Could you check a few things on this model? Use its own coordinates, in mm. A direction names the side the tool comes from. Give positions to 0.01 mm unless a question says otherwise; leave off trailing zeros. Order: outer loops, then holes, each group sorted by start corner. A loop starts at its lowest first (then second) coordinate and runs counter-clockwise, first axis right, second up. Notation, with made-up numbers: M -27.5,-3 L 2.5,-3 A22 cw 2.5,19 Z; hole C -37.5,-35.75 d11. An arc over 180 degrees is marked long. Answer in a Markdown table with one row per item. Add a question column.
```python
from build123d import *

# Parameters (mm, degrees)
F0_W      = 57.15
F0_H      = 88.9
F1_DEPTH  = 3.96875
F3_DEPTH  = 7.9375
F5_DEPTH  = 7.9375
F7_DEPTH  = 28.575
F8_R      = 9.92251
F9_DEPTH  = 25.4
F10_R     = 9.92251
F11_DEPTH = 25.4
F13_DEPTH = 7.9375
F14_R     = 10.3251
F15_DEPTH = 25.4
F16_DEPTH = 25.4
F18_DEPTH = 7.9375


with BuildPart() as f1:
    # F0 (on Front) → F1 (new body, symmetric)
    with BuildSketch(Plane.XZ):
        with Locations((28.575, 44.45)):
            Rectangle(F0_W, F0_H)
    extrude(amount=F1_DEPTH, both=True)

    # F2 (on face) → F3 (join)
    with BuildSketch(Plane(origin=(0, 0, 0), x_dir=(1, 0, 0), z_dir=(0, 0, -1))):
        with BuildLine():
            Line((0, 40.48125), (0, -3.96875))
            Line((0, -3.96875), (28.575, -3.96875))
            Line((28.575, -3.96875), (28.575, 40.48125))
            ThreePointArc((28.575, 40.48125), (14.2875, 54.76875), (0, 40.48125))
        make_face()
    extrude(amount=-F3_DEPTH)

    # F4 (on face) → F5 (join)
    with BuildSketch(Plane.XY.offset(88.9)):
        with BuildLine():
            Line((28.575, -40.160799), (28.575, 3.96875))
            Line((28.575, 3.96875), (0, 3.96875))
            Line((0, 3.96875), (0, -40.160799))
            ThreePointArc((0, -40.160799), (14.2875, -54.772343), (28.575, -40.160799))
        make_face()
    extrude(amount=-F5_DEPTH)

    # F6 (on face) → F7 (join)
    with BuildSketch(Plane(origin=(0, 0, 0), x_dir=(0, -1, 0), z_dir=(-1, 0, 0))):
        with BuildLine():
            Line((7.685762, 80.9625), (9.703519, 80.9625))
            ThreePointArc((9.703519, 80.9625), (8.694641, 81.070586), (7.685762, 80.9625))
        make_face()
        with BuildLine():
            ThreePointArc((3.96875, 76.897462), (5.179953, 79.521865), (7.685762, 80.9625))
            Line((7.685762, 80.9625), (3.96875, 80.9625))
            Line((3.96875, 80.9625), (3.96875, 76.897462))
        make_face()
        with BuildLine():
            Line((9.921576, 7.9375), (7.539107, 7.9375))
            ThreePointArc((7.539107, 7.9375), (8.730341, 7.786113), (9.921576, 7.9375))
        make_face()
        with BuildLine():
            ThreePointArc((7.539107, 7.9375), (4.993725, 9.595801), (3.96875, 12.455584))
            Line((3.96875, 12.455584), (3.96875, 7.9375))
            Line((3.96875, 7.9375), (7.539107, 7.9375))
        make_face()
    extrude(amount=-F7_DEPTH)

    # F8 (on face) → F9 (cut)
    with BuildSketch(Plane(origin=(0, 0, 0), x_dir=(1, 0, 0), z_dir=(0, 0, -1))):
        with Locations((14.2875, 40.48125)):
            Circle(F8_R)
    extrude(amount=-F9_DEPTH, mode=Mode.SUBTRACT)

    # F10 (on face) → F11 (cut)
    with BuildSketch(Plane.XY.offset(88.9)):
        with Locations((14.2875, -40.48125)):
            Circle(F10_R)
    extrude(amount=-F11_DEPTH, mode=Mode.SUBTRACT)

    # F12 (on face) → F13 (join)
    with BuildSketch(Plane(origin=(0, 3.96875, 0), x_dir=(-1, 0, 0), z_dir=(0, 1, 0))):
        with BuildLine():
            Line((-57.15, 67.517356), (-111.125, 67.517356))
            ThreePointArc((-111.125, 67.517356), (-133.35, 45.292356), (-111.125, 23.067356))
            Line((-111.125, 23.067356), (-57.15, 23.067356))
            Line((-57.15, 23.067356), (-57.15, 67.517356))
        make_face()
    extrude(amount=-F13_DEPTH)

    # F14 (on face) → F15 (cut)
    with BuildSketch(Plane.XZ.offset(3.96875)):
        with Locations((111.125, 45.292356)):
            Circle(F14_R)
        with Locations((44.45, 45.292356)):
            Circle(F14_R)
    extrude(amount=-F15_DEPTH, mode=Mode.SUBTRACT)

    # F14 (on face) → F16 (cut)
    with BuildSketch(Plane.XZ.offset(3.96875)):
        with Locations((111.125, 45.292356)):
            Circle(F14_R)
        with Locations((44.45, 45.292356)):
            Circle(F14_R)
    extrude(amount=-F16_DEPTH, mode=Mode.SUBTRACT)

    # F17 (on face) → F18 (join)
    with BuildSketch(Plane.XZ.offset(3.96875)):
        with BuildLine():
            Line((57.15, 67.517356), (57.15, 78.208678))
            ThreePointArc((57.15, 78.208678), (47.687893, 76.672868), (50.528099, 67.517356))
            Line((50.528099, 67.517356), (57.15, 67.517356))
        make_face()
        with BuildLine():
            Line((57.15, 23.067356), (51.937071, 23.067356))
            ThreePointArc((51.937071, 23.067356), (48.281511, 14.470241), (57.15, 11.533678))
            Line((57.15, 11.533678), (57.15, 23.067356))
        make_face()
    extrude(amount=-F18_DEPTH)


solid = f1.part
```
1. If I drill on line 1 along Y through (x, z) = (21, 57); line 2 along Z through (x, y) = (44.45, 2.25); line 3 along Z through (x, y) = (11.5, -52), over which ranges is the centre line in solid material (lowest first)? Write a range as [from, to].
2. For faces 1 (the flat face through (57.15, 0, 78)), 2 (the flat face through (28.575, -22, 86)), 3 (the flat face through (14, -26, 7.938)), 4 (the flat face through (85, 0, 23.067)), which set-ups out of +Z, -Z, +X, -X, +Y, -Y let a thin tool reach every point of the face, with its end or its side?
3. Will these pins go through, and if not, where does the flat tip stop? P1, Ø12.5, axis at x = 44.45, z = 45.29, coming from the -Y side; P2, Ø12, axis at x = 112.5, z = 71, coming from the -Y side; P3, Ø8.5, axis at y = 0, z = 75, coming from the +X side; P4, Ø8.5, axis at x = 85, y = 1.5, coming from the -Z side.
4. Suppose I cut it at C-C on z = 42.5. List the corners of the cut face in (x, y) for me.
5. Suppose I cut it at D-D on y = -33. List the corners of the cut face in (x, z) for me (1 decimal), plus the area to 3 significant figures.
6. Suppose I cut it at A-A on x = 44.45. List the corners of the cut face in (y, z) for me, plus the area to 3 significant figures.
7. Thinking about a two-plate mould opening in Y: for faces 5 (the flat face through (51, 3.969, 55)), 6 (the flat face through (28.575, -22, 3)), 7 (the flat face through (51, -3.969, 35)), 8 (the cylindrical face through (12.136, -30.795, 3.913)), which applies, pulls with the +Y half, pulls with the -Y half, needs draft (parallel to the pull), parting line crosses it, or undercut?
8. Suppose I cut it at B-B on y = -14. List the corners of the cut face in (x, z) for me (1 decimal).
Findings below:
| question | item | result |
|---|---|---|
| 1 | line 1 | [-3.97, 3.97] |
| 1 | line 2 | [0, 34.97], [55.62, 88.9] |
| 1 | line 3 | [0, 7.94], [80.96, 88.9] |
| 2 | face 1 | +Z, +X, +Y, -Y |
| 2 | face 2 | +Z, -Z, +X, -Y |
| 2 | face 3 | +X, -X, -Y |
| 2 | face 4 | -Z, +X, +Y, -Y |
| 3 | P1 | through |
| 3 | P2 | y = -3.97 |
| 3 | P3 | x = 57.15 |
| 3 | P4 | z = 23.07 |
| 4 | outline | M 0,-3.97 L 34.51,-3.97 L 34.51,3.97 L 0,3.97 Z; M 54.39,-3.97 L 101.18,-3.97 L 101.18,3.97 L 54.39,3.97 Z; M 121.07,-3.97 L 133.17,-3.97 L 133.17,3.97 L 121.07,3.97 Z |
| 5 | outline | M 0,0 L 7.8,0 L 7.8,7.9 L 0,7.9 Z; M 0,81 L 7.8,81 L 7.8,88.9 L 0,88.9 Z; M 20.8,0 L 28.6,0 L 28.6,7.9 L 20.8,7.9 Z; M 20.8,81 L 28.6,81 L 28.6,88.9 L 20.8,88.9 Z |
| 5 | area | 247 mm2 |
| 6 | outline | M -3.97,0 L 3.97,0 L 3.97,34.97 L -3.97,34.97 Z; M -3.97,55.62 L 3.97,55.62 L 3.97,88.9 L -3.97,88.9 Z |
| 6 | area | 542 mm2 |
| 7 | face 5 | pulls with the +Y half |
| 7 | face 6 | needs draft |
| 7 | face 7 | pulls with the -Y half |
| 7 | face 8 | undercut |
| 8 | outline | M 0,0 L 28.6,0 L 28.6,7.9 L 0,7.9 Z; M 0,81 L 28.6,81 L 28.6,88.9 L 0,88.9 Z |
